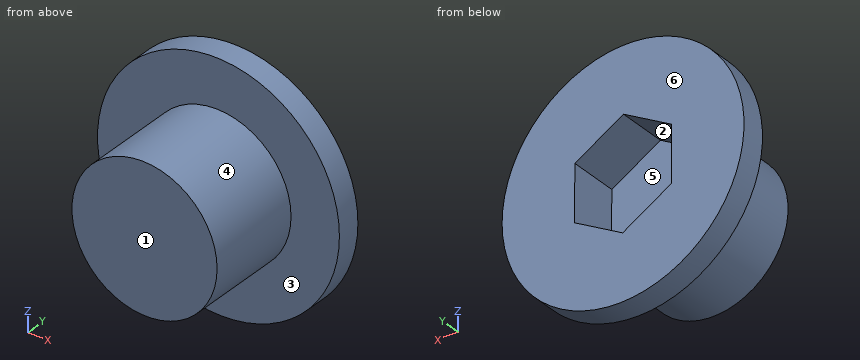
```python
from build123d import *

# Parameters (mm, degrees)
F0_R     = 7.9375
F1_DEPTH = 1.5875
F2_R     = 4.7625
F3_DEPTH = 6.35
F5_DEPTH = 3.175


with BuildPart() as f1:
    # F0 (on Front) → F1 (new body)
    with BuildSketch(Plane.XZ):
        Circle(F0_R)
    extrude(amount=F1_DEPTH)

    # F2 (on face) → F3 (join)
    with BuildSketch(Plane.XZ.offset(1.5875)):
        Circle(F2_R)
    extrude(amount=F3_DEPTH)

    # F4 (on face) → F5 (cut)
    with BuildSketch(Plane(origin=(0, 0, 0), x_dir=(-1, 0, 0), z_dir=(0, 1, 0))):
        Polygon((3.187658, 1.810987), (0.025468, 3.666086), (-3.162189, 1.855099), (-3.187658, -1.810987), (-0.025468, -3.666086), (3.162189, -1.855099), align=None)
    extrude(amount=-F5_DEPTH, mode=Mode.SUBTRACT)


solid = f1.part
```
Part model, mm, in its own coordinate system. Face numbers are marked on the shaded views. A direction names the side the tool comes from. Round coordinates to 2 decimals unless told otherwise and drop trailing zeros. Write each loop counter-clockwise with the first axis right and the second up, starting at its lowest first coordinate (ties: lowest second). Pieces come first, ordered by that corner, then holes.
Item 1: Which spindle directions (+Z, -Z, +X, -X, +Y, -Y) get a long thin tool onto all of the face, cutting with end or side? Do the marked faces 1, 2 and 3. Say none if no direction does.
Results:
face 1: +Z, -Z, +X, -X, -Y
face 2: +Y
face 3: -Y
Item 2: Cut at B-B, the plane x = -1. Give the cut face in (y, z) (1 decimal), plus the area to 3 significant figures.
Results:
outline: (-7.9, -4.7) - (-1.6, -4.7) - (-1.6, -7.9) - (0, -7.9) - (0, -3.1) - (-3.2, -3.1) - (-3.2, 3.1) - (0, 3.1) - (0, 7.9) - (-1.6, 7.9) - (-1.6, 4.7) - (-7.9, 4.7) - close
area: 64.5 mm2
Item 3: Two-plate mould, pull along X, no slides. Class the marked faces 4, 5 and 6: +X half, -X half, draft (parallel to the pull), parting line (faces both ways), or undercut.
Results:
face 4: parting line
face 5: undercut
face 6: draft
Item 4: Cut at A-A, the plane y = -2.5. Give the cut face in (x, z) (1 decimal).
Results:
outline: circle Ø9.5 at (0, 0); hole (-3.2, -1.9) - (0, -3.7) - (3.2, -1.8) - (3.2, 1.9) - (0, 3.7) - (-3.2, 1.8) - close
Item 5: Drop flat-ended pins along their axis: pin 1 Ø4 at (y, z) = (-2, -4) entering from -X; pin 2 Ø4 at (x, y) = (5.5, -1) entering from +Z; pin 3 Ø4 at (x, z) = (6, -4) entering from -Y. Give the stop position or say it passes through.
Results:
pin 1: stops at x = -7.67
pin 2: stops at z = 7.12
pin 3: stops at y = -1.59
Item 6: Cut at C-C, the plane z = -1. Give the cut face in (x, y) (1 decimal).
Results:
outline: (-7.9, -1.6) - (-4.7, -1.6) - (-4.7, -7.9) - (4.7, -7.9) - (4.7, -1.6) - (7.9, -1.6) - (7.9, 0) - (3.2, 0) - (3.2, -3.2) - (-3.2, -3.2) - (-3.2, 0) - (-7.9, 0) - close
Item 7: Probe L1, parallel to X at y = -0.5, z = -3.5; L2, parallel to Y at x = 5.25, z = -5.5; L3, parallel to Z at x = 0, y = -5.5. List the from-to ranges inside material, lowest first.
Results:
L1: x = -7.12 to -0.27, 0.31 to 7.12
L2: y = -1.59 to 0
L3: z = -4.76 to 4.76
Item 8: Cut at D-D, the plane y = -5.5. Give the cut face in (x, z) (1 decimal), plus the area to 3 significant figures.
Results:
outline: circle Ø9.5 at (0, 0)
area: 71.3 mm2
